The drawing under review shows one solid part. Ordinate dimensions are in mm from its lowest x, y, z. Round coordinates to 2 decimals unless told otherwise and drop trailing zeros. Write each loop counter-clockwise with the first axis right and the second up, starting at its lowest first coordinate (ties: lowest second). Pieces come first, ordered by that corner, then holes. Notation, with made-up numbers: M 54.5,64.5 L 108.5,64.5 A30 cw 108.5,88.5 Z; hole C 80.25,23.25 d5. An arc over 180 degrees is marked long. Write item = value, one per line. Start each with the question number.
Item 1: To check wall thickness, follow line 1 along Z through (x, y) = (51, 18.5) (1 decimal); line 2 along Z through (x, y) = (49.5, 24); line 3 along X through (y, z) = (14.5, 21). State the ranges of each line that lie inside material, in increasing order.
Item 2: Take a section at C-C, the plane x = 54.5. Give the boundary of the cut face in (y, z), plus the area to 3 significant figures.
Item 3: The part is to be moulded in two halves that separate along X. For the marked faces 1, 2 and 3, say which applies: +X half, -X half, draft (parallel to the pull), parting line (faces both ways), or undercut.
Item 4: Take a section at B-B, the plane z = 30. Give the boundary of the cut face in (x, y).
Item 5: For pin 1 Ø3 at (x, z) = (10.5, 15) entering from -Y; pin 2 Ø10 at (y, z) = (11, 27) entering from +X, all flat-tipped, find the tip position at first contact; note any pin that passes through.
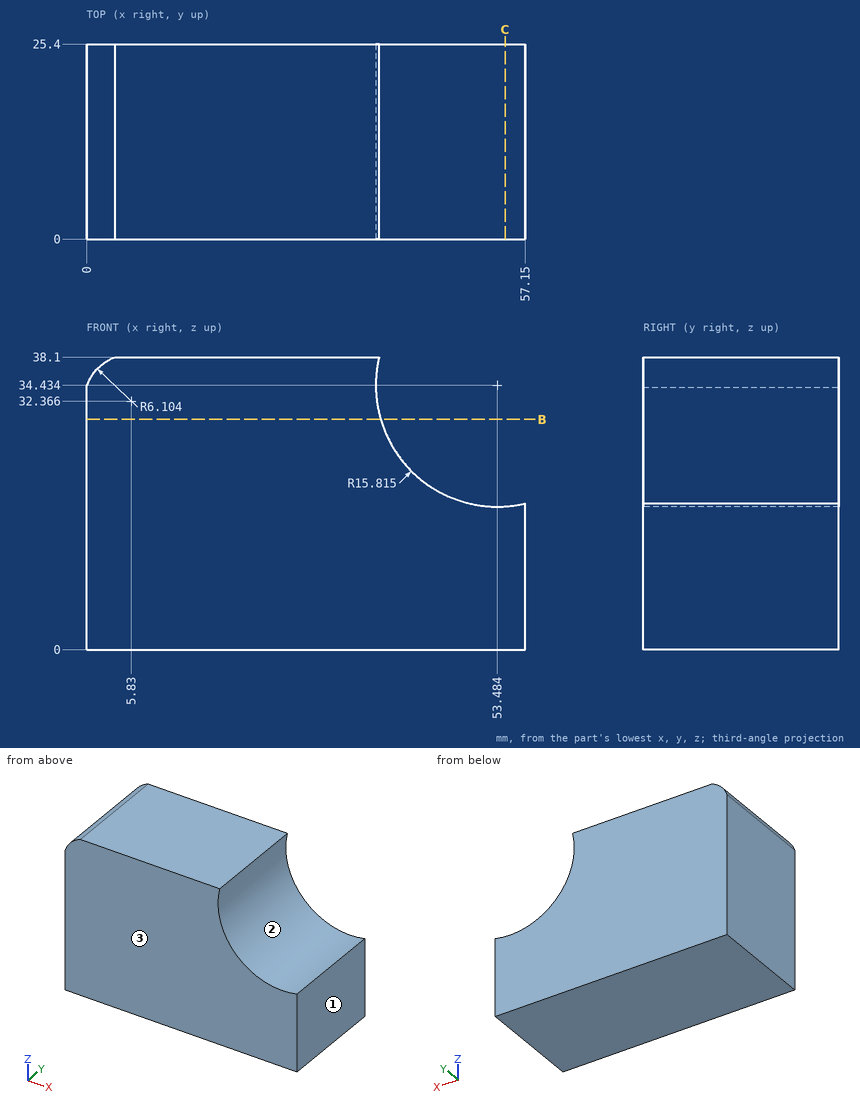
Response values:
q1.line_1 = 0 to 18.8
q1.line_2 = 0 to 19.13
q1.line_3 = 0 to 45.14
q2.outline = M 0,0 L 25.4,0 L 25.4,18.65 L 0,18.65 Z
q2.area = 474 mm2
q3.face_1 = +X half
q3.face_2 = undercut
q3.face_3 = draft
q4.outline = M 0,0 L 38.3,0 L 38.3,25.4 L 0,25.4 Z
q5.pin_1 = 0
q5.pin_2 = 43.71
